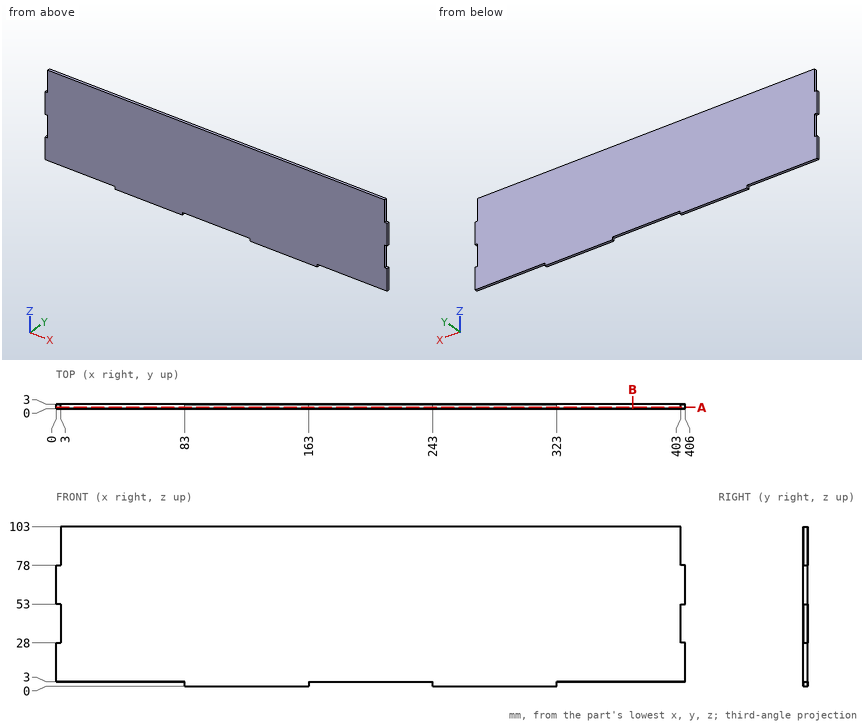
Answer from the drawing. Dimensions are ordinates in mm from the lowest x, y and z of the part. Give positions to 0.01 mm unless a question says otherwise; leave off trailing zeros. Order: outer loops, then holes, each group sorted by start corner. A loop starts at its lowest first (then second) coordinate and runs counter-clockwise, first axis right, second up. Notation, with made-up numbers: (32, -17.75) -> (70, -17.75) arc R28 ccw to (70, 9.25) -> close; hole circle Ø2 at (63, 21.5). An arc over 180 degrees is marked (long way). One line per item, written item: value.
Item 1: Straight lines are drawn through the part: probe 1 along X at (y, z) = (2.9, 92.5); probe 2 along Z at (x, y) = (370, 1.65). For each, find the intervals that lie inside material, in ascending order.
Answer sheet:
probe 1: 3 to 403
probe 2: 3 to 103
Item 2: Find section B-B, the plane x = 372. Give the vertices of the cut face in (y, z).
Answer sheet:
outline: (0, 3) -> (3, 3) -> (3, 103) -> (0, 103) -> close
Item 3: Find section A-A, the plane y = 0.85. Give the vertices of the cut face in (x, z).
Answer sheet:
outline: (0, 3) -> (83, 3) -> (83, 0) -> (163, 0) -> (163, 3) -> (243, 3) -> (243, 0) -> (323, 0) -> (323, 3) -> (406, 3) -> (406, 28) -> (403, 28) -> (403, 53) -> (406, 53) -> (406, 78) -> (403, 78) -> (403, 103) -> (3, 103) -> (3, 78) -> (0, 78) -> (0, 53) -> (3, 53) -> (3, 28) -> (0, 28) -> close
Item 4: Flat-ended cylindrical pins translate along their axes: P1, Ø12, axis at x = 46.5, z = 64, coming from the -Y side; P2, Ø0.9, axis at y = 1.5, z = 2, coming from the -X side; P3, Ø1.5, axis at y = 1.5, z = 2, coming from the +X side; P4, Ø0.9, axis at x = 53.5, y = 1, coming from the -Z side. Find the tip coordinate at first contact, or state that the pin passes through.
Answer sheet:
P1: y = 0
P2: x = 83
P3: x = 323
P4: z = 3
